Here's how the part is built. I have some questions about the finished solid (model axes, mm). Face numbers are marked on the shaded views. A direction names the side the tool comes from. Round coordinates to 2 decimals unless told otherwise and drop trailing zeros. Write each loop counter-clockwise with the first axis right and the second up, starting at its lowest first coordinate (ties: lowest second). Pieces come first, ordered by that corner, then holes. Notation, with made-up numbers: (71.5, -26) - (95.5, -26) arc R5 cw to (95.5, -20) - close; hole circle Ø11 at (80.5, 31.5). An arc over 180 degrees is marked (long way). Write item = value, one per line. Start each with the question number.
Item 1: For P1, Ø6, axis at x = 4, z = -25.5, coming from the +Y side; P2, Ø3, axis at y = 69.5, z = 4.5, coming from the -X side; P3, Ø11.5, axis at y = 43, z = -36, coming from the -X side; P4, Ø3.5, axis at x = -2, z = 36, coming from the +Y side, each with a flat end and sliding along its axis, tell me the tip position at first contact or that it passes through.
Item 2: If we section it at A-A (z = -45.97): Please give me the cut outline in (x, y) (3 decimals).
Item 3: Thinking about a two-plate mould opening in Z: for the marked faces 4, 5 and 6, which applies, pulls with the +Z half, pulls with the -Z half, needs draft (parallel to the pull), parting line crosses it, or undercut?
Item 4: Which directions (+Z, -Z, +X, -X, +Y, -Y) give clear straight access to the entire face, cutting with the end or side of a thin tool? Please do the marked faces 1, 2 and 3.
Item 5: If I drill on line 1 along Z through (x, y) = (-5, 7); line 2 along Z through (x, y) = (11.5, 48.5); line 3 along Y through (x, z) = (-4.5, -45.97), over which ranges is the centre line in solid material (lowest first)? Write a range as [from, to].
Item 6: If we section it at C-C (y = 7.62): Give the number of separate pieces and of enclosed holes in the cut face, and give its area (3 significant figures).
Item 7: If we section it at B-B (x = 7.5): Please give me the cut outline in (y, z), and give its area (3 significant figures).
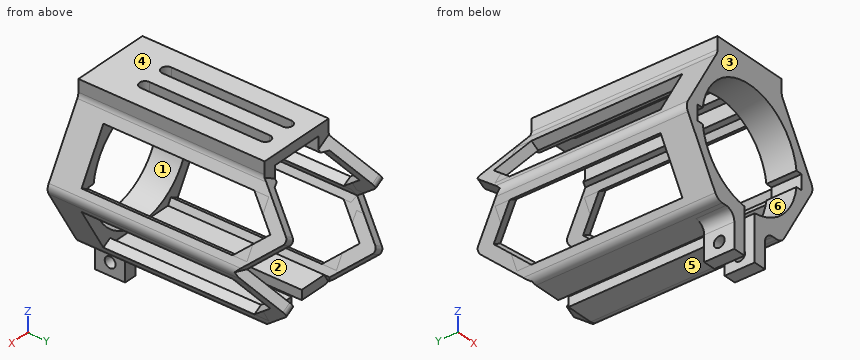
```python
from build123d import *

# Parameters (mm, degrees)
BOSS_EXTRUDE1_DEPTH  = 114.3
SKETCH2_W            = 6.35
SKETCH2_H            = 17.78
CUT_EXTRUDE2_DEPTH   = 99.06
SKETCH3_W            = 27.183356596
SKETCH3_H            = 83.82
CUT_EXTRUDE3_DEPTH   = 99.06
SKETCH4_W            = 27.183356596
SKETCH4_H            = 83.82
CUT_EXTRUDE4_DEPTH   = 99.06
SKETCH7_W            = 3.263536018
SKETCH7_H            = 7.713600016
CUT_EXTRUDE7_DEPTH   = 15.24
CUT_EXTRUDE8_DEPTH   = 99.06
SKETCH10_W           = 39.883356596
SKETCH10_H           = 114.3
BOSS_EXTRUDE2_DEPTH  = 7.62
CUT_EXTRUDE11_DEPTH  = 81.28
BOSS_EXTRUDE9_DEPTH  = 4.826
MIRROR9_COPY_1_DEPTH = 4.826
MIRROR9_COPY_2_DEPTH = 4.826
CUT_EXTRUDE13_DEPTH  = 19.941678176
CUT_EXTRUDE14_DEPTH  = 19.941678176
SKETCH17_W           = 27.183356538
SKETCH17_H           = 4.826
CUT_EXTRUDE15_DEPTH  = 99.06
SKETCH18_W           = 39.883356596
SKETCH18_H           = 7.62
CUT_EXTRUDE16_DEPTH  = 19.941678176
CUT_EXTRUDE18_DEPTH  = 19.941678176
SKETCH20_W           = 27.183356538
SKETCH20_H           = 2.54
CUT_EXTRUDE19_DEPTH  = 79.118321824
FILLET1_R            = 5.08
FILLET2_R            = 2.54
SKETCH21_R           = 2.749999961
CUT_EXTRUDE20_DEPTH  = 79.118321824


with BuildPart() as part:
    # Sketch1 → Boss-Extrude1 (new body)
    with BuildSketch(Plane(origin=(0, 0, 0), x_dir=(1, 0, 0), z_dir=(0, 1, 0))):
        with BuildLine():
            Line((39.883356596, 0), (19.941678298, 34.54))
            Line((19.941678298, 34.54), (9.525, 34.54))
            Line((9.525, 34.54), (9.525, 52.32))
            Line((9.525, 52.32), (3.175, 52.32))
            Line((3.175, 52.32), (3.175, 34.54))
            Line((3.175, 34.54), (3.175, 29.28841025))
            ThreePointArc((3.175, 29.28841025), (0, -29.46), (-3.175, 29.28841025))
            Line((-3.175, 29.28841025), (-3.175, 34.54))
            Line((-3.175, 34.54), (-3.175, 52.32))
            Line((-3.175, 52.32), (-9.525, 52.32))
            Line((-9.525, 52.32), (-9.525, 34.54))
            Line((-9.525, 34.54), (-19.941678298, 34.54))
            Line((-19.941678298, 34.54), (-39.883356596, 0))
            Line((-39.883356596, 0), (-19.941678298, -34.54))
            Line((-19.941678298, -34.54), (19.941678298, -34.54))
            Line((19.941678298, -34.54), (39.883356596, 0))
        make_face()
    extrude(amount=BOSS_EXTRUDE1_DEPTH)

    # Sketch2 → Cut-Extrude2 (cut)
    with BuildSketch(Plane(origin=(0, 114.3, 0), x_dir=(1, 0, 0), z_dir=(0, 1, 0))):
        with Locations((-6.35, 43.43)):
            Rectangle(SKETCH2_W, SKETCH2_H)
        with Locations((6.35, 43.43)):
            Rectangle(SKETCH2_W, SKETCH2_H)
    extrude(amount=-CUT_EXTRUDE2_DEPTH, mode=Mode.SUBTRACT)

    # Sketch3 → Cut-Extrude3 (cut)
    with BuildSketch(Plane(origin=(-29.912517447, 0, -17.27), x_dir=(-0.49999999999999617, 0, 0.8660254037844409), z_dir=(-0.8660254037844408, 0, -0.4999999999999961))):
        with Locations((0, 57.15)):
            Rectangle(SKETCH3_W, SKETCH3_H)
    extrude(amount=-CUT_EXTRUDE3_DEPTH, mode=Mode.SUBTRACT)

    # Sketch4 → Cut-Extrude4 (cut)
    with BuildSketch(Plane(origin=(29.912517447, 0, -17.27), x_dir=(-0.500000000000004, 0, -0.8660254037844364), z_dir=(0.8660254037844365, 0, -0.500000000000004))):
        with Locations((0, 57.15)):
            Rectangle(SKETCH4_W, SKETCH4_H)
    extrude(amount=-CUT_EXTRUDE4_DEPTH, mode=Mode.SUBTRACT)

    # Sketch7 → Cut-Extrude7 (cut)
    with BuildSketch(Plane.XZ):
        with Locations((-30.838217531, 0)):
            Rectangle(SKETCH7_W, SKETCH7_H)
        with Locations((30.838217531, 0)):
            Rectangle(SKETCH7_W, SKETCH7_H)
    extrude(amount=-CUT_EXTRUDE7_DEPTH, mode=Mode.SUBTRACT)

    # Sketch8 → Cut-Extrude8 (cut)
    with BuildSketch(Plane(origin=(0, 114.3, 0), x_dir=(1, 0, 0), z_dir=(0, 1, 0))):
        Polygon((-3.175, 29.714), (3.175, 29.714), (17.155385899, 29.714), (34.310771797, 0), (17.155385899, -29.714), (-17.155385899, -29.714), (-34.310771797, 0), (-17.155385899, 29.714), align=None)
    extrude(amount=-CUT_EXTRUDE8_DEPTH, mode=Mode.SUBTRACT)

    # Sketch10 → Boss-Extrude2 (add)
    with BuildSketch(Plane.XY.offset(34.54)):
        with Locations((0, 57.15)):
            Rectangle(SKETCH10_W, SKETCH10_H)
    extrude(amount=BOSS_EXTRUDE2_DEPTH)

    # Sketch12 → Cut-Extrude11 (cut)
    with BuildSketch(Plane(origin=(-29.912517447, 0, -17.27), x_dir=(-0.4999999999999998, 0, 0.8660254037844388), z_dir=(-0.8660254037844388, 0, -0.4999999999999998))):
        Polygon((19.941678298, 114.3), (0, 114.3), (19.941678298, 94.358321702), align=None)
        Polygon((-19.941678298, 94.358321702), (0, 114.3), (-19.941678298, 114.3), align=None)
        Polygon((6.259743879, 99.06), (0, 105.319743879), (-6.259743879, 99.06), align=None)
    cut_extrude11 = extrude(amount=-CUT_EXTRUDE11_DEPTH, mode=Mode.SUBTRACT)

    # Mirror2: Cut-Extrude11 across plane
    add(cut_extrude11.mirror(Plane(origin=(0, 0, 0), x_dir=(0, 0, 1), z_dir=(1, 0, 0))), mode=Mode.SUBTRACT)

    # Sketch11 → Boss-Extrude9 (add)
    with BuildSketch(Plane(origin=(-29.912517447, 0, -17.27), x_dir=(-0.4999999999999998, 0, 0.8660254037844388), z_dir=(-0.8660254037844388, 0, -0.4999999999999998))):
        Polygon((-13.591678298, 91.728065581), (0, 105.319743879), (13.591678298, 91.728065581), (19.941678298, 94.358321702), (0, 114.3), (-19.941678298, 94.358321702), align=None)
    boss_extrude9 = extrude(amount=-BOSS_EXTRUDE9_DEPTH)

    # Mirror8: Boss-Extrude9 across plane
    add(boss_extrude9.mirror(Plane.XY))

    # Mirror9 copy 1 sketch → Mirror9 copy 1 (add)
    with BuildSketch(Plane(origin=(29.912517447, 0, 17.27), x_dir=(0.4999999999999998, 0, -0.8660254037844388), z_dir=(0.8660254037844388, 0, 0.4999999999999998))):
        Polygon((-13.591678298, 91.728065581), (0, 105.319743879), (13.591678298, 91.728065581), (19.941678298, 94.358321702), (0, 114.3), (-19.941678298, 94.358321702), align=None)
    extrude(amount=-MIRROR9_COPY_1_DEPTH)

    # Mirror9 copy 2 sketch → Mirror9 copy 2 (add)
    with BuildSketch(Plane(origin=(29.912517447, 0, -17.27), x_dir=(0.4999999999999998, 0, 0.8660254037844388), z_dir=(0.8660254037844388, 0, -0.4999999999999998))):
        Polygon((-13.591678298, -91.728065581), (0, -105.319743879), (13.591678298, -91.728065581), (19.941678298, -94.358321702), (0, -114.3), (-19.941678298, -94.358321702), align=None)
    extrude(amount=-MIRROR9_COPY_2_DEPTH)

    # Sketch15 → Cut-Extrude13 (cut)
    with BuildSketch(Plane(origin=(0, 114.3, 0), x_dir=(1, 0, 0), z_dir=(0, 1, 0))):
        Polygon((-17.155385899, 29.714), (-19.941678298, 34.54), (19.941678298, 34.54), (17.155385899, 29.714), align=None)
    extrude(amount=-CUT_EXTRUDE13_DEPTH, mode=Mode.SUBTRACT)

    # Sketch16 → Cut-Extrude14 (cut)
    with BuildSketch(Plane(origin=(0, 114.3, 0), x_dir=(1, 0, 0), z_dir=(0, 1, 0))):
        Polygon((-19.941678298, -34.54), (19.941678298, -34.54), (11.5828011, -29.714), (-11.5828011, -29.714), align=None)
    extrude(amount=-CUT_EXTRUDE14_DEPTH, mode=Mode.SUBTRACT)

    # Sketch17 → Cut-Extrude15 (cut)
    with BuildSketch(Plane(origin=(0, 114.3, 0), x_dir=(1, 0, 0), z_dir=(0, 1, 0))):
        with Locations((0, -32.127)):
            Rectangle(SKETCH17_W, SKETCH17_H)
    extrude(amount=-CUT_EXTRUDE15_DEPTH, mode=Mode.SUBTRACT)

    # Sketch18 → Cut-Extrude16 (cut)
    with BuildSketch(Plane(origin=(0, 114.3, 0), x_dir=(1, 0, 0), z_dir=(0, 1, 0))):
        with Locations((0, -38.35)):
            Rectangle(SKETCH18_W, SKETCH18_H)
    extrude(amount=-CUT_EXTRUDE16_DEPTH, mode=Mode.SUBTRACT)

    # Sketch19 → Cut-Extrude18 (cut)
    with BuildSketch(Plane.XY.offset(42.16)):
        with BuildLine():
            Line((-9.545839134, 23.07), (-9.545839134, 83.988321824))
            ThreePointArc((-9.545839134, 83.988321824), (-6.795839134, 86.738321824), (-4.045839134, 83.988321824))
            Line((-4.045839134, 83.988321824), (-4.045839134, 23.07))
            ThreePointArc((-4.045839134, 23.07), (-6.795839134, 20.32), (-9.545839134, 23.07))
        make_face()
        with BuildLine():
            Line((9.545839134, 23.07), (9.545839134, 83.988321824))
            ThreePointArc((9.545839134, 83.988321824), (6.795839134, 86.738321824), (4.045839134, 83.988321824))
            Line((4.045839134, 83.988321824), (4.045839134, 23.07))
            ThreePointArc((4.045839134, 23.07), (6.795839134, 20.32), (9.545839134, 23.07))
        make_face()
    extrude(amount=-CUT_EXTRUDE18_DEPTH, mode=Mode.SUBTRACT)

    # Sketch20 → Cut-Extrude19 (cut)
    with BuildSketch(Plane(origin=(0, 94.358321824, 0), x_dir=(1, 0, 0), z_dir=(0, 1, 0))):
        with Locations((0, -35.81)):
            Rectangle(SKETCH20_W, SKETCH20_H)
    extrude(amount=-CUT_EXTRUDE19_DEPTH, mode=Mode.SUBTRACT)

    # Fillet1
    fillet1_edges = [part.edges().sort_by_distance(p)[0] for p in [
        (19.941678298, 47.179160851, 34.54),
        (-39.883356596, 47.179160851, 0),
        (-19.941678298, 47.179160851, -34.54),
        (39.883356596, 47.179160851, 0),
        (-19.941678298, 47.179160851, 34.54),
        (19.941678298, 47.179160851, -34.54),
        (-9.525, 7.62, -34.54),
        (9.525, 7.62, -34.54),
    ]]
    fillet(fillet1_edges, radius=FILLET1_R)

    # Fillet2
    fillet2_edges = [part.edges().sort_by_distance(p)[0] for p in [
        (27.822798147, 114.3, 16.0635),
        (-27.822798147, 114.3, -16.0635),
        (-27.822798147, 114.3, 16.0635),
        (27.822798147, 114.3, -16.0635),
    ]]
    fillet(fillet2_edges, radius=FILLET2_R)

    # Sketch21 → Cut-Extrude20 (cut)
    with BuildSketch(Plane(origin=(9.525, 0, 0), x_dir=(0, 0, -1), z_dir=(1, 0, 0))):
        with Locations((45.97, 7.62)):
            Circle(SKETCH21_R)
    extrude(amount=-CUT_EXTRUDE20_DEPTH, mode=Mode.SUBTRACT)


solid = part.part
```
Reply:
q1.P1 = through
q1.P2 = -38.15
q1.P3 = -22.42
q1.P4 = 94.36
q2.outline = (-9.525, 0) - (-3.175, 0) - (-3.175, 4.87) - (-9.525, 4.87) - close; (-9.525, 10.37) - (-3.175, 10.37) - (-3.175, 15.24) - (-9.525, 15.24) - close; (3.175, 0) - (9.525, 0) - (9.525, 4.87) - (3.175, 4.87) - close; (3.175, 10.37) - (9.525, 10.37) - (9.525, 15.24) - (3.175, 15.24) - close
q3.face_4 = pulls with the +Z half
q3.face_5 = pulls with the -Z half
q3.face_6 = undercut
q4.face_1 = +Y, -Y
q4.face_2 = +Y
q4.face_3 = +Z, -Z, +X, -X, -Y
q5.line_1 = [-52.32, -48.65], [-43.29, -29.03], [29.03, 42.16]
q5.line_2 = [-34.54, -29.71], [37.08, 42.16]
q5.line_3 = [0, 4.87], [10.37, 15.24]
q6.separate_pieces = 3
q6.enclosed_holes = 0
q6.area = 1,790 mm2
q7.outline = (0, -52.32) - (15.24, -52.32) - (15.24, -34.54) - (94.36, -34.54) - (94.36, -29.71) - (15.24, -29.71) - (15.24, -28.49) - (0, -28.49) - close; (0, 28.49) - (15.24, 28.49) - (15.24, 37.08) - (20.41, 37.08) - (20.41, 42.16) - (0, 42.16) - close; (86.65, 37.08) - (94.36, 37.08) - (94.36, 42.16) - (86.65, 42.16) - close; hole circle Ø5.5 at (7.62, -45.97)
q7.area = 995 mm2
